Autodesk Inventor part; units mm, degrees
ref_plane "YZ Plane" through (0, 0, 0) normal (1, 0, 0) x (0, 1, 0)
ref_plane "XZ Plane" through (0, 0, 0) normal (0, 1, 0) x (-1, 0, 0)
ref_plane "XY Plane" through (0, 0, 0) normal (0, 0, 1) x (1, 0, 0)
sketch "Skizze1" plane through (0, 0, 0) normal (1, 0, 0) x (0, 1, 0)
  line L0 (0, 0) -> (7, 0)
  line L1 (7, 0) -> (7, 7)
  line L2 (7, 7) -> (0, 7)
  line L3 (0, 7) -> (0, 0)
  line L4 (3, 7) -> (4, 7)
  line L5 (4, 7) -> (4, 6.7)
  line L6 (4, 6.7) -> (3, 6.7)
  line L7 (3, 6.7) -> (3, 7)
  line L8 (3, 0.3) -> (4, 0.3)
  line L9 (4, 0.3) -> (4, 0)
  line L10 (4, 0) -> (3, 0)
  line L11 (3, 0) -> (3, 0.3)
  dimension "d0" = 7
  dimension "d1" = 7
  dimension "d2" = 1
  dimension "d3" = 0.3
  dimension "d5" = 3
extrude "Extrusion1" add sketch "Skizze1" along normal blind 6 contours L3 L2 L7 L6 L5 L1 L0 L9 L8 L11
sketch "Skizze2" plane through (6, 0, 0) normal (1, 0, 0) x (0, 0, -1)
  line L0 (0, 7) -> (-7, 7)
  line L1 (-7, 7) -> (-7, 4)
  line L2 (-7, 0) -> (0, 0)
  line L3 (0, 0) -> (0, 3)
  line L4 (-6.5, 6.5) -> (-0.5, 6.5)
  line L5 (-0.5, 6.5) -> (-0.5, 0.5)
  line L6 (-0.5, 0.5) -> (-6.5, 0.5)
  line L7 (-6.5, 0.5) -> (-6.5, 6.5)
  dimension "d8" = 0.5
  dimension "d9" = 0.5
  dimension "d10" = 0.5
  dimension "d11" = 0.5
extrude "Extrusion2" cut sketch "Skizze2" against normal blind 1.1
sketch "Skizze3" plane through (0, 0, 0) normal (-1, 0, 0) x (0, 0, 1)
  line L0 (7, 0) -> (0, 0)
  line L1 (0, 4) -> (0, 7)
  line L2 (1.98, 5.02) -> (2.48, 5.02)
  line L3 (2.48, 5.02) -> (2.48, 4.52)
  line L4 (2.48, 4.52) -> (1.98, 4.52)
  line L5 (1.98, 4.52) -> (1.98, 5.02)
  line L6 (4.52, 5.02) -> (5.02, 5.02)
  line L7 (5.02, 5.02) -> (5.02, 4.52)
  line L8 (5.02, 4.52) -> (4.52, 4.52)
  line L9 (4.52, 4.52) -> (4.52, 5.02)
  line L10 (1.98, 1.98) -> (2.48, 1.98)
  line L11 (2.48, 1.98) -> (2.48, 2.48)
  line L12 (2.48, 2.48) -> (1.98, 2.48)
  line L13 (1.98, 2.48) -> (1.98, 1.98)
  line L14 (4.52, 1.98) -> (5.02, 1.98)
  line L15 (5.02, 1.98) -> (5.02, 2.48)
  line L16 (5.02, 2.48) -> (4.52, 2.48)
  line L17 (4.52, 2.48) -> (4.52, 1.98)
  dimension "d14" = 0.5
  dimension "d15" = 0.5
  dimension "d16" = 0.5
  dimension "d17" = 0.5
  dimension "d18" = 0.5
  dimension "d19" = 0.5
  dimension "d20" = 0.5
  dimension "d21" = 0.5
  dimension "d24" = 1.98
  dimension "d25" = 3.04
  dimension "d26" = 3.04
  dimension "d27" = 1.98
extrude "Extrusion3" add sketch "Skizze3" along normal blind 6
sketch "Skizze4" plane through (4.9, 0, 0) normal (1, 0, 0) x (0, 0, -1)
  line L0 (-6.5, 0.5) -> (-6.5, 6.5)
  line L1 (-0.5, 0.5) -> (-6.5, 0.5)
  line L2 (-0.5, 6.5) -> (-0.5, 0.5)
  circle A0 centre (-4.9, 3.5) radius 0.9
  circle A1 centre (-2.1, 3.5) radius 0.9
  line L3 (-4.9, 3.5) -> (-2.1, 3.5)
  line L4 (-6.5, 6.5) -> (-0.5, 6.5)
  point P0 (0, 0)
  dimension "d30" = 1.8
  dimension "d31" = 1.8
  dimension "d32" = 2.8
  dimension "d33" = 3
  dimension "d34" = 1.6
extrude "Extrusion4" add sketch "Skizze4" along normal blind 0.2 contours A0 | A1
properties part number "cny-70"
Verification items for the finished model (mm, model axes). A direction names the side the tool comes from. Coordinates: 2 decimals unless noted, no trailing zeros. Loops run counter-clockwise (first coordinate to the right, second up) from the corner with the lowest first, then second, coordinate; pieces in that order, holes last. Notation, with made-up numbers: (39, -38.75) -> (70, -38.75) arc R12 cw to (70, -22.75) -> close; hole circle Ø6 at (79.5, 32). An arc over 180 degrees is marked (long way). Answer in a Markdown table with one row per item.
1) Draft check along Y on faces 1 (the face through (3, 6, 7)), 2 (the face through (3, 7, 3)), 3 (the face through (5.5, 3.5, 0.5)). Enter one of: released by +Y, released by -Y, zero draft, split by the parting line, or undercut.
The answers:
| item | result |
|---|---|
| face 1 | zero draft |
| face 2 | released by +Y |
| face 3 | undercut |
2) Depth check by flat-ended pin: P1, Ø0.6, axis at x = -3, z = 2, coming from the -Y side; P2, Ø0.9, axis at y = 3.5, z = 4.5, coming from the +X side; P3, Ø0.6, axis at x = -1.5, y = 2, coming from the -Z side. Enter the tip coordinate at first touch or a pass-through.
The answers:
| item | result |
|---|---|
| P1 | stops at y = 1.98 |
| P2 | stops at x = 5.1 |
| P3 | stops at z = 1.98 |
3) Section check D-D (y = 3.5). Record the cut outline in (x, z), and give its area (3 significant figures).
The answers:
| item | result |
|---|---|
| outline | (0, 0.3) -> (6, 0.3) -> (6, 0.5) -> (4.9, 0.5) -> (4.9, 1.2) -> (5.1, 1.2) -> (5.1, 3) -> (4.9, 3) -> (4.9, 4) -> (5.1, 4) -> (5.1, 5.8) -> (4.9, 5.8) -> (4.9, 6.5) -> (6, 6.5) -> (6, 6.7) -> (0, 6.7) -> close |
| area | 32.5 mm2 |
4) Section check A-A (x = -5). Record the cut outline in (y, z), and give its area (3 significant figures).
The answers:
| item | result |
|---|---|
| outline | (1.98, 1.98) -> (2.48, 1.98) -> (2.48, 2.48) -> (1.98, 2.48) -> close; (1.98, 4.52) -> (2.48, 4.52) -> (2.48, 5.02) -> (1.98, 5.02) -> close; (4.52, 1.98) -> (5.02, 1.98) -> (5.02, 2.48) -> (4.52, 2.48) -> close; (4.52, 4.52) -> (5.02, 4.52) -> (5.02, 5.02) -> (4.52, 5.02) -> close |
| area | 1.00 mm2 |
5) Access from +Z, -Z, +X, -X, +Y, -Y to the whole of each face (thin tool, end or side, straight path). Record for faces 4 (the face through (3, 3.5, 0.3)), 5 (the face through (5.1, 4, 5)), 6 (the face through (3, 3.5, 6.7)).
The answers:
| item | result |
|---|---|
| face 4 | -Z, +X, -X |
| face 5 | +X |
| face 6 | +Z, +X, -X |
6) Section check B-B (y = 2.25). Record the cut outline in (x, z), and give its area (3 significant figures).
The answers:
| item | result |
|---|---|
| outline | (-6, 1.98) -> (0, 1.98) -> (0, 0) -> (6, 0) -> (6, 0.5) -> (4.9, 0.5) -> (4.9, 6.5) -> (6, 6.5) -> (6, 7) -> (0, 7) -> (0, 5.02) -> (-6, 5.02) -> (-6, 4.52) -> (0, 4.52) -> (0, 2.48) -> (-6, 2.48) -> close |
| area | 41.4 mm2 |
7) Scan lines: line 1 along Z through (x, y) = (5.75, 1.75); line 2 along Y through (x, z) = (5, 5.5). Record each from-to range of solid material in increasing order. Write a range as from..to.
The answers:
| item | result |
|---|---|
| line 1 | z = 0..0.5, 6.5..7 |
| line 2 | y = 0..0.5, 2.83..4.17, 6.5..7 |
8) Section check C-C (z = 5.25). Record the cut outline in (x, y).
The answers:
| item | result |
|---|---|
| outline | (0, 0) -> (6, 0) -> (6, 0.5) -> (4.9, 0.5) -> (4.9, 2.67) -> (5.1, 2.67) -> (5.1, 4.33) -> (4.9, 4.33) -> (4.9, 6.5) -> (6, 6.5) -> (6, 7) -> (0, 7) -> close |
